Geometry: final body of the model. Coordinates: model frame, mm. Give positions to 0.01 mm unless a question says otherwise; leave off trailing zeros. Order: outer loops, then holes, each group sorted by start corner. A loop starts at its lowest first (then second) coordinate and runs counter-clockwise, first axis right, second up. Notation, with made-up numbers: (-17, 53.5) - (18, 53.5) arc R15 cw to (18, 74.5) - close; hole circle Ø3 at (72, -34.5). An arc over 180 degrees is marked (long way). Put each result on its own line as item: value. Start each with the question number.
1. Section C-C on y = 29. Return the cut outline in (x, z), plus the area to 3 significant figures.
2. Section B-B on x = 0. Return the cut outline in (y, z).
3. First-contact query: P1, Ø1, axis at y = -25.5, z = -3.5, coming from the -X side; P2, Ø5, axis at x = -4, z = -3.5, coming from the +Y side; P3, Ø5, axis at y = 19, z = 5, coming from the -X side; P4, Ø3.5, axis at y = 0, z = 0, coming from the -X side. Flat tips, straight axial feed; report the tip coordinate or a pass-through.
4. Section A-A on z = -2.75. Return the cut outline in (x, y).
5. Section D-D on x = 26. Return the cut outline in (y, z), plus the area to 3 significant figures.
6. Mould query, pull axis Y, two halves, no side actions, for faces 1 (the cylindrical face through (-23.623, 21.207, 3.121)), 2 (the cylindrical face through (-0.34, 31.95, 1.55)), 3 (the cylindrical face through (-24.503, -23.572, 0.089)). Classes: pulls with the +Y half, pulls with the -Y half, needs draft (parallel to the pull), parting line crosses it, or undercut.
7. Ray query, line 1 along X through (y, z) = (0, 4.25); line 2 along Z through (x, y) = (31.9, 0); line 3 along Y through (x, z) = (-23, -3.5). Return the intervals inside material, ascending. Write a range as from..to.
from build123d import *

# Parameters (mm, degrees)
CROQUIS1_R                   = 30
SALIENTE_EXTRUIR1_DEPTH      = 6.35
SALIENTE_EXTRUIR1_DEPTH_BACK = 6.35
CROQUIS3_R                   = 1.5875
CORTAR_EXTRUIR1_DEPTH        = 35
CORTAR_EXTRUIR1_DEPTH_BACK   = 35
CROQUIS4_R                   = 1.5875
CORTAR_EXTRUIR2_DEPTH        = 35.0000001
CORTAR_EXTRUIR2_DEPTH_BACK   = 35.0000001
CROQUIS5_R                   = 1.75
CORTAR_EXTRUIR3_DEPTH        = 82.485020219


with BuildPart() as part:
    # Croquis1 → Saliente-Extruir1 (new body, two sides)
    with BuildSketch(Plane.XY) as saliente_extruir1_sk:
        with BuildLine():
            Line((-19.128482186, 28.108738308), (-28.108738308, 19.128482186))
            ThreePointArc((-28.108738308, 19.128482186), (-24.04163056, -24.04163056), (19.128482186, -28.108738308))
            Line((19.128482186, -28.108738308), (28.108738308, -19.128482186))
            ThreePointArc((28.108738308, -19.128482186), (24.04163056, 24.04163056), (-19.128482186, 28.108738308))
        make_face()
        Circle(CROQUIS1_R, mode=Mode.SUBTRACT)
    extrude(amount=SALIENTE_EXTRUIR1_DEPTH)
    extrude(saliente_extruir1_sk.sketch, amount=-SALIENTE_EXTRUIR1_DEPTH_BACK)

    # Croquis3 → Cortar-Extruir1 (cut, two sides)
    with BuildSketch(Plane(origin=(0, 0, 0), x_dir=(1, 0, 0), z_dir=(0, 1, 0))) as cortar_extruir1_sk:
        Circle(CROQUIS3_R)
    extrude(amount=CORTAR_EXTRUIR1_DEPTH, mode=Mode.SUBTRACT)
    extrude(cortar_extruir1_sk.sketch, amount=-CORTAR_EXTRUIR1_DEPTH_BACK, mode=Mode.SUBTRACT)

    # Croquis4 → Cortar-Extruir2 (cut, two sides)
    with BuildSketch(Plane(origin=(0, 0, 0), x_dir=(0, 0, -1), z_dir=(1, 0, 0))) as cortar_extruir2_sk:
        Circle(CROQUIS4_R)
    extrude(amount=CORTAR_EXTRUIR2_DEPTH, mode=Mode.SUBTRACT)
    extrude(cortar_extruir2_sk.sketch, amount=-CORTAR_EXTRUIR2_DEPTH_BACK, mode=Mode.SUBTRACT)

    # Croquis5 → Cortar-Extruir3 (cut, through all)
    with BuildSketch(Plane(origin=(-23.618610247, 23.618610247, 0), x_dir=(0, 0, 1), z_dir=(-0.707106781, 0.707106781, 0))):
        with Locations((-3.5, 0)):
            Circle(CROQUIS5_R)
        with Locations((3.5, 0)):
            Circle(CROQUIS5_R)
    extrude(amount=-CORTAR_EXTRUIR3_DEPTH, mode=Mode.SUBTRACT)


solid = part.part
Resolved:
1. outline: (-17.75, -6.35) - (-7.68, -6.35) - (-7.68, 6.35) - (-17.75, 6.35) - close; (7.68, -6.35) - (17.75, -6.35) - (17.75, 6.35) - (7.68, 6.35) - close
1. area: 256 mm^2
2. outline: (-34, -6.35) - (-30, -6.35) - (-30, -1.59) - (-34, -1.59) - close; (-34, 1.59) - (-30, 1.59) - (-30, 6.35) - (-34, 6.35) - close; (30, -6.35) - (34, -6.35) - (34, -1.59) - (30, -1.59) - close; (30, 1.59) - (34, 1.59) - (34, 6.35) - (30, 6.35) - close
3. P1: x = -23.04
3. P2: y = 33.97
3. P3: x = -29.73
3. P4: x = -34
4. outline: (-28.11, 19.13) arc R34 ccw to (19.13, -28.11) - (22.5, -24.74) - (20.07, -22.3) arc R30 cw to (-22.3, 20.07) - (-24.74, 22.5) - close; (-22.5, 24.74) - (-20.07, 22.3) arc R30 cw to (22.3, -20.07) - (24.74, -22.5) - (28.11, -19.13) arc R34 ccw to (-19.13, 28.11) - close
5. outline: (-21.24, -6.35) - (-14.97, -6.35) - (-14.97, 6.35) - (-21.24, 6.35) - close; (14.97, -6.35) - (21.91, -6.35) - (21.91, 6.35) - (14.97, 6.35) - close
5. area: 168 mm^2
6. face 1: undercut
6. face 2: needs draft
6. face 3: parting line crosses it
7. line 1: -34..-30, 30..34
7. line 2: -6.35..-1.59, 1.59..6.35
7. line 3: -25.04..-19.26, 19.26..20.53
